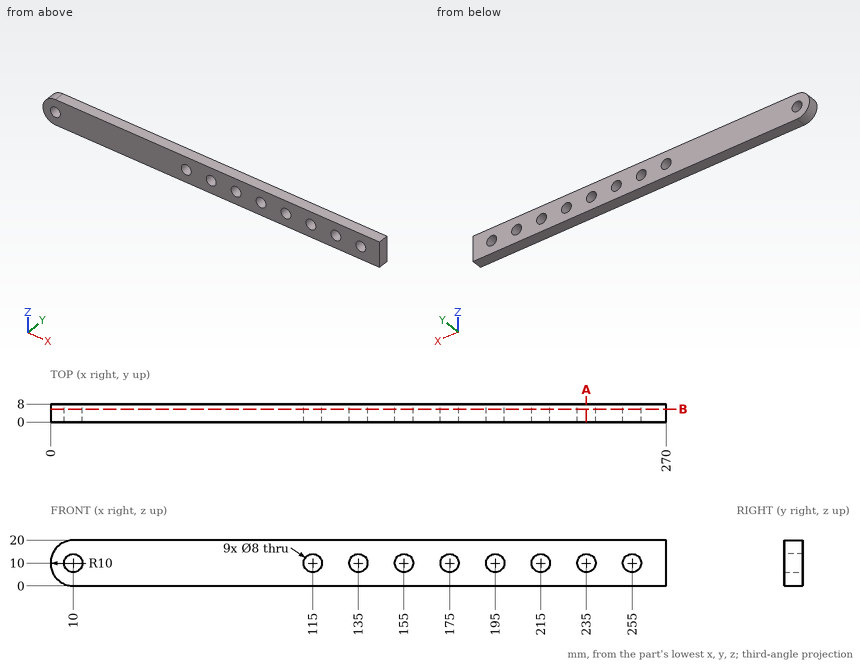
Geometry check sheet. Reference: drawing and pictorial views, mm from the part's lowest x, y, z. Give positions to 0.01 mm unless a question says otherwise; leave off trailing zeros. Loops run counter-clockwise (first coordinate to the right, second up) from the corner with the lowest first, then second, coordinate; pieces in that order, holes last. Notation, with made-up numbers: (37.5, 77) -> (55.5, 77) arc R20 ccw to (55.5, 116) -> close; hole circle Ø8 at (70.25, 19.25). An arc over 180 degrees is marked (long way). Answer in a Markdown table with one row per item. Add a question column.
1) Cross-section at B-B on y = 5.75. State how many separate pieces and enclosed holes the cut face has, and give its area (3 significant figures).
2) Cross-section at A-A on x = 235. Record the boundary of the cut face in (y, z).
3) Material ranges on probe 1 along Z at (x, y) = (135, 3.5); probe 2 along Z at (x, y) = (234, 5); probe 3 along X at (y, z) = (6, 18.25), recorded low to high. Write a range as from..to.
Outcome:
| question | item | result |
|---|---|---|
| 1 | separate pieces | 1 |
| 1 | enclosed holes | 9 |
| 1 | area | 4,900 mm^2 |
| 2 | outline | (0, 0) -> (8, 0) -> (8, 6) -> (0, 6) -> close; (0, 14) -> (8, 14) -> (8, 20) -> (0, 20) -> close |
| 3 | probe 1 | z = 0..6, 14..20 |
| 3 | probe 2 | z = 0..6.13, 13.87..20 |
| 3 | probe 3 | x = 4.35..270 |
